```python
from build123d import *

# Parameters (mm, degrees)
SKETCH1_R                           = 15.875
BOSS_EXTRUDE1_DEPTH                 = 6.35
SKETCH2_R                           = 6.35
CUT_EXTRUDE1_DEPTH                  = 24.3313898
TAP_DRILL_FOR_2_56_TAP2_D           = 1.778
TAP_DRILL_FOR_2_56_TAP2_CSINK_D     = 3.048
TAP_DRILL_FOR_2_56_TAP2_CSINK_ANGLE = 100
CIRPATTERN1_COUNT                   = 2
CIRPATTERN2_COUNT                   = 2
SKETCH11_R                          = 2.286
CUT_EXTRUDE2_DEPTH                  = 24.3313898
CIRPATTERN3_COUNT                   = 2
CUT_EXTRUDE3_DEPTH                  = 24.3313898


with BuildPart() as part:
    # Sketch1 → Boss-Extrude1 (new body)
    with BuildSketch(Plane(origin=(0, 0, 0), x_dir=(1, 0, 0), z_dir=(0, 1, 0))):
        with Locations(Location((0, 0, 0), (0, 0, 270))):
            Circle(SKETCH1_R)
    extrude(amount=BOSS_EXTRUDE1_DEPTH)

    # Sketch2 → Cut-Extrude1 (cut, through all)
    with BuildSketch(Plane(origin=(0, 6.35, 0), x_dir=(1, 0, 0), z_dir=(0, 1, 0))):
        with Locations(Location((0, 0, 0), (0, 0, 270))):
            Circle(SKETCH2_R)
    extrude(amount=-CUT_EXTRUDE1_DEPTH, mode=Mode.SUBTRACT)

    # Tap Drill for #2-56 Tap2 (through all)
    with Locations(Plane(origin=(0, 6.35, 0), x_dir=(1, 0, 0), z_dir=(0, 1, 0))):
        with Locations((0, 11.1252)):
            tap_drill_for_2_56_tap2 = CounterSinkHole(TAP_DRILL_FOR_2_56_TAP2_D / 2, TAP_DRILL_FOR_2_56_TAP2_CSINK_D / 2, counter_sink_angle=TAP_DRILL_FOR_2_56_TAP2_CSINK_ANGLE)

    # CirPattern1: Tap Drill for #2-56 Tap2 ×2 about axis
    cirpattern1_axis = Axis((0, 0, 0), (0, 1, 0))
    for i in range(1, CIRPATTERN1_COUNT):
        add(tap_drill_for_2_56_tap2.rotate(cirpattern1_axis, i * 360 / CIRPATTERN1_COUNT), mode=Mode.SUBTRACT)

    # Sketch10 → Tap Drill for #2-56 Tap1 (revolve, cut)
    with BuildSketch(Plane(origin=(11.1252, 6.35, 0), x_dir=(0, 0, 1), z_dir=(1, 0, 0))):
        Polygon((0, 0), (0, 4.34416509), (0.889, 3.81), (0.889, 0.532828266), (1.524, 0), align=None)
    tap_drill_for_2_56_tap1 = revolve(axis=Axis((11.1252, 12.7, 0), (0, -1, 0)), mode=Mode.SUBTRACT)

    # CirPattern2: Tap Drill for #2-56 Tap1 ×2 about axis
    cirpattern2_axis = Axis((0, 0, 0), (0, 1, 0))
    for i in range(1, CIRPATTERN2_COUNT):
        add(tap_drill_for_2_56_tap1.rotate(cirpattern2_axis, i * 360 / CIRPATTERN2_COUNT), mode=Mode.SUBTRACT)

    # Sketch11 → Cut-Extrude2 (cut, through all)
    with BuildSketch(Plane(origin=(0, 6.35, 0), x_dir=(1, 0, 0), z_dir=(0, 1, 0))):
        with Locations(Location((8.328911597, 7.35641814, 0), (0, 0, 270))):
            Circle(SKETCH11_R)
    cut_extrude2 = extrude(amount=-CUT_EXTRUDE2_DEPTH, mode=Mode.SUBTRACT)

    # CirPattern3: Cut-Extrude2 ×2 about axis
    cirpattern3_axis = Axis((0, 0, 0), (0, 1, 0))
    for i in range(1, CIRPATTERN3_COUNT):
        add(cut_extrude2.rotate(cirpattern3_axis, i * 360 / CIRPATTERN3_COUNT), mode=Mode.SUBTRACT)

    # Sketch12 → Cut-Extrude3 (cut, through all)
    with BuildSketch(Plane(origin=(0, 6.35, 0), x_dir=(1, 0, 0), z_dir=(0, 1, 0))):
        with BuildLine():
            Line((-6.39758264, 4.883452605), (-4.554151289, 6.87011727))
            ThreePointArc((-4.554151289, 6.87011727), (-4.0916663, 6.887412726), (-4.074370844, 6.424927737))
            Line((-4.074370844, 6.424927737), (-5.917802195, 4.438263073))
            ThreePointArc((-5.917802195, 4.438263073), (-6.380287183, 4.420967617), (-6.39758264, 4.883452605))
        make_face()
    extrude(amount=-CUT_EXTRUDE3_DEPTH, mode=Mode.SUBTRACT)


solid = part.part
```
Part model, mm, in its own coordinate system. A direction names the side the tool comes from. Round coordinates to 2 decimals unless told otherwise and drop trailing zeros. Loops run counter-clockwise (first coordinate to the right, second up) from the corner with the lowest first, then second, coordinate; pieces in that order, holes last.
1. 3-axis set-ups, long thin cutter, end or side, ignore diameter. For faces 5 (the face through (-11.914, 4.202, -0.41)), 6 (the face through (-4.98, 3.22, -5.45)), 7 (the face through (0, 6.35, 7)): which of +Z, -Z, +X, -X, +Y, -Y reach the whole face in a straight line?
Solutions:
face 5: +Y
face 6: +Y, -Y
face 7: +Z, -Z, +X, -X, +Y
2. Drill centre lines: line 1 along X through (y, z) = (3.9, 0) (3 decimals); line 2 along Z through (x, y) = (-0.5, 0.5); line 3 along Z through (x, y) = (-4.5, 3.5). Where is each one in solid material? Low to high.
Solutions:
line 1: x = -15.875 to -12.014, -10.236 to -6.35, 6.35 to 10.236, 12.014 to 15.875
line 2: z = -15.87 to -11.86, -10.39 to -6.33, 6.33 to 10.39, 11.86 to 15.87
line 3: z = -15.22 to -6.92, -5.97 to -4.48, 4.48 to 15.22
3. Flat gauge pins, fed straight in: pin 1 (1.6 mm diameter, centred on x = 0, z = -11.13, fed in from -Y); pin 2 (1.6 mm diameter, centred on x = 11.13, z = 0, fed in from +Y); pin 3 (1.5 mm diameter, centred on y = 2, z = -8.5, fed in from +X). Where does each tip first touch, or does it go through?
Solutions:
pin 1: passes through
pin 2: stops at y = 2.49
pin 3: stops at x = 13.85
4. Slice it at B-B (x = 7). Give the cut face in (y, z), and give its area (3 significant figures).
Solutions:
outline: (0, -14.25) - (6.35, -14.25) - (6.35, -9.22) - (0, -9.22) - close; (0, -5.5) - (6.35, -5.5) - (6.35, 14.25) - (0, 14.25) - close
area: 157 mm2
5. Slice it at C-C (z = -9). Give the cut face in (x, y), and give its area (3 significant figures).
Solutions:
outline: (-13.08, 0) - (6.74, 0) - (6.74, 6.35) - (-13.08, 6.35) - close; (9.92, 0) - (13.08, 0) - (13.08, 6.35) - (9.92, 6.35) - close
area: 146 mm2
6. Two-plate mould, pull along X, no slides. Class faces 1 (the face through (-5.49, 3.22, -5.86)), 2 (the face through (10.26, 3.22, -6.13)), 3 (the face through (0, 0, 7)), 4 (the face through (-15.497, 3.131, -3.441)): pulls with the +X half, pulls with the -X half, needs draft (parallel to the pull), parting line crosses it, or undercut.
Solutions:
face 1: undercut
face 2: undercut
face 3: needs draft
face 4: parting line crosses it
7. Slice it at A-A (x = 0). Give the cut face in (y, z) (3 decimals), and give its area (3 significant figures).
Solutions:
outline: (0, -15.875) - (6.35, -15.875) - (6.35, -12.649) - (5.817, -12.014) - (0, -12.014) - close; (0, -10.236) - (5.817, -10.236) - (6.35, -9.601) - (6.35, -6.35) - (0, -6.35) - close; (0, 6.35) - (6.35, 6.35) - (6.35, 9.601) - (5.817, 10.236) - (0, 10.236) - close; (0, 12.014) - (5.817, 12.014) - (6.35, 12.649) - (6.35, 15.875) - (0, 15.875) - close
area: 97.7 mm2
8. Slice it at D-D (y = 4). Count the separate pieces of the cut face and the enclosed holes in it, and give its area (3 significant figures).
Solutions:
separate pieces: 1
enclosed holes: 8
area: 620 mm2
